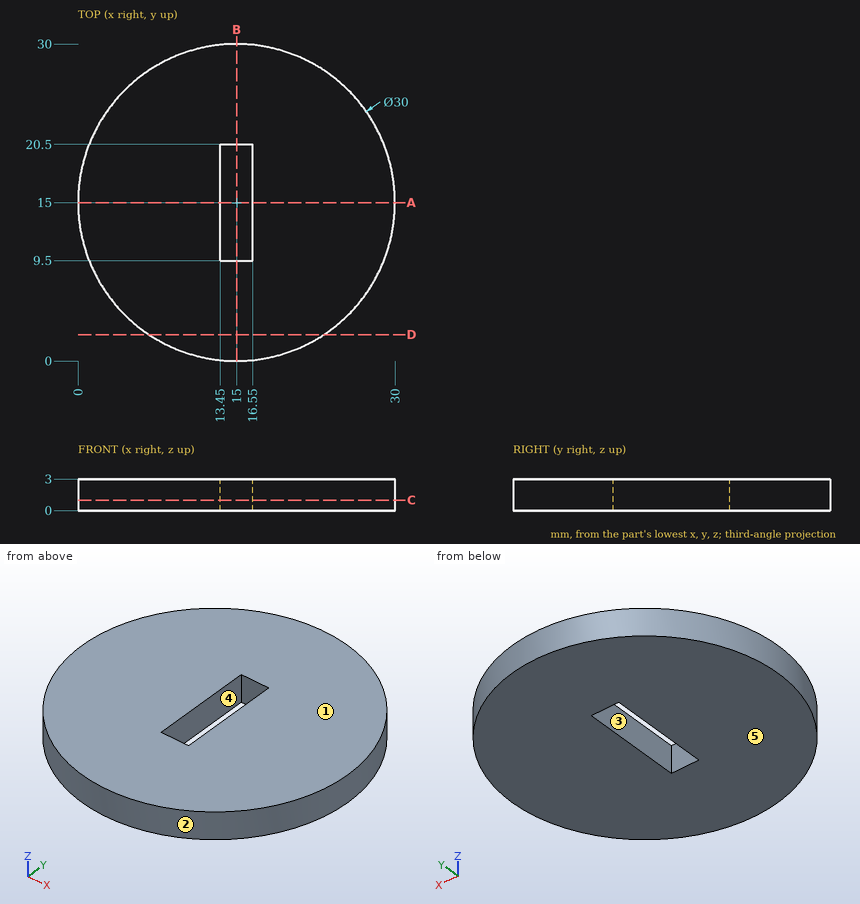
Source: three-view drawing plus pictorial views. Frame: mm from the lowest corner of the part. A direction names the side the tool comes from. Round coordinates to 2 decimals unless told otherwise and drop trailing zeros. Write each loop counter-clockwise with the first axis right and the second up, starting at its lowest first coordinate (ties: lowest second). Pieces come first, ordered by that corner, then holes. Notation, with made-up numbers: M 29,33 L 51,33 A24 ccw 51,45 Z; hole C 36,43.25 d10. An arc over 180 degrees is marked long. Write item = value, one per line.
Item 1: Pin query (flat end, axial travel): P1, Ø1, axis at x = 11.5, z = 2, coming from the -Y side; P2, Ø0.9, axis at y = 13.5, z = 1, coming from the -X side; P3, Ø1, axis at x = 23, y = 4, coming from the -Z side. Return the tip coordinate at first contact, or that it passes through.
Findings:
P1 = 0.3
P2 = 0.04
P3 = 0
Item 2: Material intervals for line 1 along X through (y, z) = (14.75, 2); line 2 along X through (y, z) = (12.5, 2.05); line 3 along Y through (x, z) = (14.5, 2.45), sorted ascending. Write a range as [from, to].
Findings:
line_1 = [0, 13.45], [16.55, 30]
line_2 = [0.21, 13.45], [16.55, 29.79]
line_3 = [0.01, 9.5], [20.5, 29.99]
Item 3: Section query C-C on z = 1. Return loops of the section in (x, y), then the cut area to 3 significant figures.
Findings:
outline = C 15,15 d30; hole M 13.45,9.5 L 16.55,9.5 L 16.55,20.5 L 13.45,20.5 Z
area = 673 mm^2
Item 4: Section query A-A on y = 15. Return loops of the section in (x, z).
Findings:
outline = M 0,0 L 13.45,0 L 13.45,3 L 0,3 Z; M 16.55,0 L 30,0 L 30,3 L 16.55,3 Z
Item 5: Access query for the marked faces 4 and 5. Directions: +Z, -Z, +X, -X, +Y, -Y. A direction counts if a zero-diameter tool reaches every point of the face in a straight line with its end or side. Return the directions, or none.
Findings:
face_4 = +Z, -Z
face_5 = -Z, +X, -X, +Y, -Y
Item 6: Section query B-B on x = 15. Return loops of the section in (y, z).
Findings:
outline = M 0,0 L 9.5,0 L 9.5,3 L 0,3 Z; M 20.5,0 L 30,0 L 30,3 L 20.5,3 Z
Item 7: Pull-direction query (Y, two-part tool) for the marked faces 1, 2 and 3; classes: pulls with the +Y half, pulls with the -Y half, needs draft (parallel to the pull), parting line crosses it, or undercut.
Findings:
face_1 = needs draft
face_2 = parting line crosses it
face_3 = undercut
Item 8: Section query D-D on y = 2.5. Return loops of the section in (x, z), then the cut area to 3 significant figures.
Findings:
outline = M 6.71,0 L 23.29,0 L 23.29,3 L 6.71,3 Z
area = 49.7 mm^2
